Verification items for the finished model (mm, model axes). A direction names the side the tool comes from. Give positions to 0.01 mm unless a question says otherwise; leave off trailing zeros. Order: outer loops, then holes, each group sorted by start corner. A loop starts at its lowest first (then second) coordinate and runs counter-clockwise, first axis right, second up. Notation, with made-up numbers: (10, -39.5) - (20, -39.5) arc R15 cw to (20, -26.5) - close; hole circle Ø1 at (72, 45). An arc over 180 degrees is marked (long way). Answer as a JSON object with one key per item and string values. Group by question number.
(1) Access from +Z, -Z, +X, -X, +Y, -Y to the whole of each face (thin tool, end or side, straight path). Record for faces 1 (the face through (14, -11.049, 0)), 2 (the face through (5.78, -2.78, -12.54)), 3 (the face through (2.82, -10.8, -8.28)), 4 (the face through (0.405, 4.167, 1.312)), 5 (the face through (15.74, -0.18, 13.54)).
(2) Section check B-B (x = 1.5). Record the boundary of the cut face in (y, z).
(3) Section check A-A (x = 9.75). Record the boundary of the cut face in (y, z).
(4) Thickness scan on line 1 (X direction, y = -11.75, z = -0.75); line 2 (Z direction, x = 5.75, y = -8); line 3 (Z direction, x = 2.25, y = 0.5). Record the ranges inside material, lowest first.
(5) Depth check by flat-ended pin: pin 1 Ø2.5 at (x, z) = (12.5, 1.5) entering from +Y; pin 2 Ø2.5 at (x, z) = (13, 1.5) entering from -Y; pin 3 Ø5 at (x, y) = (12, 7.5) entering from -Z. Enter the tip coordinate at first touch or a pass-through.
(6) Mould release check, pull along Y, two halves, no side actions. Record for faces 6 (the face through (14, 11.049, 0)), 7 (the face through (8.12, -0.997, -4.488)), 8 (the face through (9.819, -1.844, 14.046)): +Y half, -Y half, draft (parallel to the pull), parting line (faces both ways), or undercut.
Autodesk Inventor part; units mm, degrees
ref_plane "cut1_XY" through (15.875, 11.049, 0) normal (1, 0, 0) x (0, 0, -1)
ref_plane "cut1_YZ" through (15.875, 11.049, 0) normal (0, 0, -1) x (0, 1, 0)
ref_plane "cut1_ZX" through (15.875, 11.049, 0) normal (0, 1, 0) x (1, 0, 0)
sketch "Sketch_1" plane through (0, 0, 0) normal (0, 0, 1) x (1, 0, 0)
  line L0 (15.875, 0) -> (0, 0)
  line L1 (0, 0) -> (0, 12.846)
  line L2 (0, 12.846) -> (0.762, 13.6081)
  line L3 (0.762, 13.6081) -> (4.826, 13.6081)
  line L4 (4.826, 13.6081) -> (5.588, 12.846)
  line L5 (5.588, 12.846) -> (6.35, 12.846)
  line L6 (6.35, 12.846) -> (6.35, 14.1669)
  line L7 (6.35, 14.1669) -> (15.113, 14.1669)
  line L8 (15.113, 14.1669) -> (15.875, 13.4049)
  line L9 (15.875, 13.4049) -> (15.875, 0)
  line L10 (15.875, 0) -> (0, 0)
revolve "Revolution1" add sketch "Sketch_1" angle 360 about axis through (15.875, 0, 0) along (1, 0, 0)
sketch "Sketch_6" plane through (0, 0, 0) normal (0, 0, 1) x (1, 0, 0)
  line L0 (15.875, 0) -> (0, 0)
  line L1 (0, 0) -> (0, 4.3688)
  line L2 (0, 4.3688) -> (0.7987, 4.3688)
  line L3 (0.7987, 4.3688) -> (15.24, 4.8197)
  line L4 (15.24, 4.8197) -> (15.875, 5.4547)
  line L5 (15.875, 5.4547) -> (15.875, 0)
  line L6 (15.875, 0) -> (0, 0)
revolve "Revolution2" cut sketch "Sketch_6" angle 360 about axis through (15.875, 0, 0) along (1, 0, 0)
thread "Thread1"
sketch "Sketch_5" plane through (15.875, 0, 0) normal (1, 0, 0) x (0, 0, -1)
  line L0 (-56.6674, -28.3337) -> (56.6674, -28.3337)
  line L1 (56.6674, -28.3337) -> (56.6674, 28.3337)
  line L2 (56.6674, 28.3337) -> (-56.6674, 28.3337)
  line L3 (-56.6674, 28.3337) -> (-56.6674, -28.3337)
  line L4 (-28.3337, -11.049) -> (28.3337, -11.049)
  line L5 (28.3337, -11.049) -> (28.3337, 11.049)
  line L6 (28.3337, 11.049) -> (-28.3337, 11.049)
  line L7 (-28.3337, 11.049) -> (-28.3337, -11.049)
extrude "Extrusion1" cut sketch "Sketch_5" against normal blind 4.7752
sketch "Sketch_24" plane through (0, 0, 0) normal (0, 0, 1) x (1, 0, 0)
  line L0 (6.35, 0) -> (5.588, 0)
  line L1 (5.429, 14.1669) -> (5.429, 14.0827)
  line L2 (5.429, 14.0827) -> (6.2275, 13.2842)
  arc A0 (6.2275, 13.1046) -> (6.2275, 13.2842) centre (6.1377, 13.1944) ccw
  line L3 (6.2275, 13.1046) -> (5.969, 12.846)
  line L4 (5.969, 12.846) -> (5.588, 12.846)
  line L5 (5.588, 12.846) -> (5.588, 12.5921)
  line L6 (5.588, 12.5921) -> (6.35, 12.5921)
  line L7 (6.35, 12.5921) -> (6.35, 13.449)
  line L8 (6.35, 13.449) -> (5.6322, 14.1669)
  line L9 (5.6322, 14.1669) -> (5.429, 14.1669)
revolve "Revolution3" add sketch "Sketch_24" angle 360 about axis through (6.35, 0, 0) along (1, 0, 0)
ref_plane "cut1_XY" through (15.875, 11.049, 0) normal (1, 0, 0) x (0, 0, -1)
ref_plane "cut1_YZ" through (15.875, 11.049, 0) normal (0, 0, -1) x (0, 1, 0)
ref_plane "cut1_ZX" through (15.875, 11.049, 0) normal (0, 1, 0) x (1, 0, 0)
ref_plane "cut2_XY" through (15.875, -11.049, 0) normal (1, 0, 0) x (0, 0, -1)
ref_plane "cut2_YZ" through (15.875, -11.049, 0) normal (0, 0, -1) x (0, 1, 0)
ref_plane "cut2_ZX" through (15.875, -11.049, 0) normal (0, 1, 0) x (1, 0, 0)
ref_plane "cutf1_XY" through (15.875, 0, 0) normal (0, 0, 1) x (1, 0, 0)
ref_plane "cutf1_YZ" through (15.875, 0, 0) normal (1, 0, 0) x (0, 1, 0)
ref_plane "cutf1_ZX" through (15.875, 0, 0) normal (0, 1, 0) x (0, 0, 1)
ref_plane "cutf2_XY" through (11.0998, 0, 0) normal (0, 0, 1) x (1, 0, 0)
ref_plane "cutf2_YZ" through (11.0998, 0, 0) normal (1, 0, 0) x (0, 1, 0)
ref_plane "cutf2_ZX" through (11.0998, 0, 0) normal (0, 1, 0) x (0, 0, 1)
ref_plane "lovra_XY" through (15.875, 0, 0) normal (1, 0, 0) x (0, 1, 0)
ref_plane "lovra_YZ" through (15.875, 0, 0) normal (0, 1, 0) x (0, 0, 1)
ref_plane "lovra_ZX" through (15.875, 0, 0) normal (0, 0, 1) x (1, 0, 0)
ref_plane "lovra1_XY" through (11.0998, 0, 0) normal (1, 0, 0) x (0, 0, -1)
ref_plane "lovra1_YZ" through (11.0998, 0, 0) normal (0, 0, -1) x (0, 1, 0)
ref_plane "lovra1_ZX" through (11.0998, 0, 0) normal (0, 1, 0) x (1, 0, 0)
ref_plane "lovra2_XY" through (11.0998, 11.049, 0) normal (1, 0, 0) x (0, 0, -1)
ref_plane "lovra2_YZ" through (11.0998, 11.049, 0) normal (0, 0, -1) x (0, 1, 0)
ref_plane "lovra2_ZX" through (11.0998, 11.049, 0) normal (0, 1, 0) x (1, 0, 0)
ref_plane "lovra21_XY" through (0, 0, 5.2705) normal (1, 0, 0) x (0, 0, -1)
ref_plane "lovra21_YZ" through (0, 0, 5.2705) normal (0, 0, -1) x (0, 1, 0)
ref_plane "lovra21_ZX" through (0, 0, 5.2705) normal (0, 1, 0) x (1, 0, 0)
ref_plane "lovra22_XY" through (0, 0, -5.2705) normal (1, 0, 0) x (0, 0, -1)
ref_plane "lovra22_YZ" through (0, 0, -5.2705) normal (0, 0, -1) x (0, 1, 0)
ref_plane "lovra22_ZX" through (0, 0, -5.2705) normal (0, 1, 0) x (1, 0, 0)
ref_plane "lovra3_XY" through (11.0998, -11.049, 0) normal (1, 0, 0) x (0, 0, -1)
ref_plane "lovra3_YZ" through (11.0998, -11.049, 0) normal (0, 0, -1) x (0, 1, 0)
ref_plane "lovra3_ZX" through (11.0998, -11.049, 0) normal (0, 1, 0) x (1, 0, 0)
ref_plane "olen_XY" through (15.875, 0, 0) normal (1, 0, 0) x (0, 0, -1)
ref_plane "olen_YZ" through (15.875, 0, 0) normal (0, 0, -1) x (0, 1, 0)
ref_plane "olen_ZX" through (15.875, 0, 0) normal (0, 1, 0) x (1, 0, 0)
ref_plane "to_mounting_bracket_XY" through (22.225, 0, 0) normal (1, 0, 0) x (0, 0, -1)
ref_plane "to_mounting_bracket_YZ" through (22.225, 0, 0) normal (0, 0, -1) x (0, 1, 0)
ref_plane "to_mounting_bracket_ZX" through (22.225, 0, 0) normal (0, 1, 0) x (1, 0, 0)
ref_plane "to_nut_XY" through (0, 0, 0) normal (1, 0, 0) x (0, 0, -1)
ref_plane "to_nut_YZ" through (0, 0, 0) normal (0, 0, -1) x (0, 1, 0)
ref_plane "to_nut_ZX" through (0, 0, 0) normal (0, 1, 0) x (1, 0, 0)
ref_plane "to_pin_XY" through (30.9626, 0, 0) normal (0, 0, 1) x (1, 0, 0)
ref_plane "to_pin_YZ" through (30.9626, 0, 0) normal (1, 0, 0) x (0, 1, 0)
ref_plane "to_pin_ZX" through (30.9626, 0, 0) normal (0, 1, 0) x (0, 0, 1)
ref_plane "to_screw_XY" through (15.0876, 10.2743, -7.0612) normal (0, 1, 0) x (1, 0, 0)
ref_plane "to_screw_YZ" through (15.0876, 10.2743, -7.0612) normal (1, 0, 0) x (0, 0, -1)
ref_plane "to_screw_ZX" through (15.0876, 10.2743, -7.0612) normal (0, 0, -1) x (0, 1, 0)
ref_plane "to_tube_XY" through (5.588, 0, 0) normal (1, 0, 0) x (0, 0, -1)
ref_plane "to_tube_YZ" through (5.588, 0, 0) normal (0, 0, -1) x (0, 1, 0)
ref_plane "to_tube_ZX" through (5.588, 0, 0) normal (0, 1, 0) x (1, 0, 0)
properties part number "090000_rear_head"
Solutions:
{
 "1": {"face 1": "+Z, -Z, +X, -Y", "face 2": "none", "face 3": "-X", "face 4": "+X, -X", "face 5": "+Z, +X"},
 "2": {"outline": "circle Ø27.22 at (0, 0); hole circle Ø8.78 at (0, 0)"},
 "3": {"outline": "circle Ø28.33 at (0, 0); hole circle Ø9.3 at (0, 0)"},
 "4": {"line 1": "x = 0 to 11.1", "line 2": "z = -11.55 to -11.2, -10.05 to 10.05, 11.2 to 11.55", "line 3": "z = -13.6 to -4.39, 4.39 to 13.6"},
 "5": {"pin 1": "stops at y = 11.05", "pin 2": "stops at y = -11.05", "pin 3": "stops at z = -13.26"},
 "6": {"face 6": "+Y half", "face 7": "undercut", "face 8": "parting line"}
}
